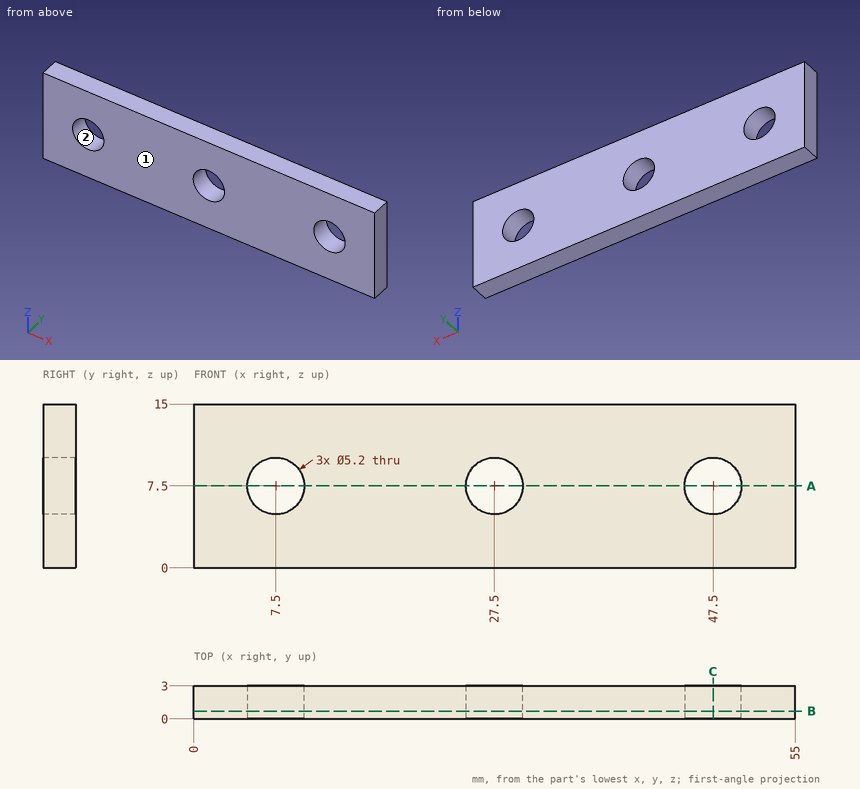
The figure shows three views and two pictorial views of one solid part (mm, origin at its lowest corner). Answer the questions. Coordinates: 2 decimals unless noted, no trailing zeros. Loops run counter-clockwise (first coordinate to the right, second up) from the corner with the lowest first, then second, coordinate; pieces in that order, holes last. Notation, with made-up numbers: (47.5, 67.25) -> (70.5, 67.25) arc R9 ccw to (70.5, 73.25) -> close; hole circle Ø3 at (53.25, 68). An arc over 180 degrees is marked (long way). Write item = value, one per line. Start each with the question number.
1) A cutting plane is placed at B-B (y = 0.7). Give the vertices of the cut face in (x, z).
2) The mould has two halves that part along Z. Classify the marked faces 1 and 2: released by +Z, released by -Z, zero draft, split by the parting line, or undercut.
3) Given pin 1 Ø3 at (x, z) = (27.5, 7.5) entering from +Y, flat-ended and moving along its own axis, determine where the tip first touches the part or whether it passes through.
4) Straight lines are drawn through the part: line 1 (X direction, y = 2, z = 7.5); line 2 (Z direction, x = 27.5, y = 1.05); line 3 (Z direction, x = 29.5, y = 1.95). For each, find the intervals that lie inside material, in ascending order. Write a range as from..to.
5) A cutting plane is placed at C-C (x = 47.5). Give the vertices of the cut face in (y, z), then the cut area to 3 significant figures.
6) A cutting plane is placed at A-A (z = 7.5). Give the vertices of the cut face in (x, y), then the cut area to 3 significant figures.
Responses:
q1.outline = (0, 0) -> (55, 0) -> (55, 15) -> (0, 15) -> close; hole circle Ø5.2 at (7.5, 7.5); hole circle Ø5.2 at (27.5, 7.5); hole circle Ø5.2 at (47.5, 7.5)
q2.face_1 = zero draft
q2.face_2 = undercut
q3.pin_1 = through
q4.line_1 = 0..4.9, 10.1..24.9, 30.1..44.9, 50.1..55
q4.line_2 = 0..4.9, 10.1..15
q4.line_3 = 0..5.84, 9.16..15
q5.outline = (0, 0) -> (3, 0) -> (3, 4.9) -> (0, 4.9) -> close; (0, 10.1) -> (3, 10.1) -> (3, 15) -> (0, 15) -> close
q5.area = 29.4 mm²
q6.outline = (0, 0) -> (4.9, 0) -> (4.9, 3) -> (0, 3) -> close; (10.1, 0) -> (24.9, 0) -> (24.9, 3) -> (10.1, 3) -> close; (30.1, 0) -> (44.9, 0) -> (44.9, 3) -> (30.1, 3) -> close; (50.1, 0) -> (55, 0) -> (55, 3) -> (50.1, 3) -> close
q6.area = 118 mm²
